Check sheet for the modelled part. Datum: model origin and axes. Units: mm. Face numbers are marked on the shaded views. Give positions to 0.01 mm unless a question says otherwise; leave off trailing zeros. Loops run counter-clockwise (first coordinate to the right, second up) from the corner with the lowest first, then second, coordinate; pieces in that order, holes last.
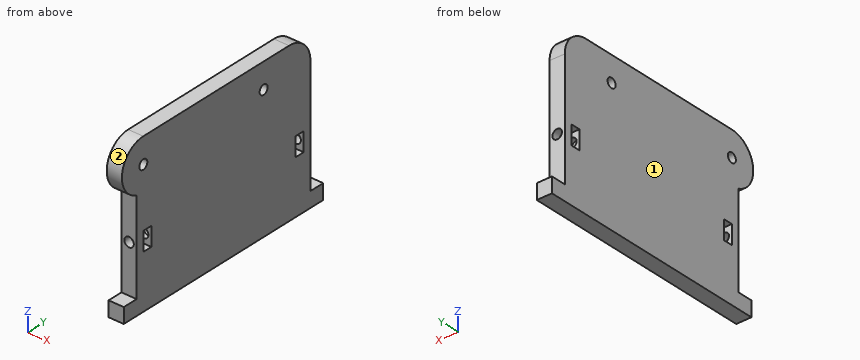
Autodesk Fusion 360 part; units mm, degrees
sketch "Sketch1" plane through (0, 0, 0) normal (1, 0, 0) x (0, 1, 0)
  line L0 (-32.5, 4.8) -> (-37.3, 4.8)
  line L1 (-37.3, 4.8) -> (-37.3, 0)
  line L2 (-37.3, 0) -> (37.3, 0)
  line L3 (37.3, 0) -> (37.3, 4.8)
  line L4 (37.3, 4.8) -> (32.5, 4.8)
  line L5 (-32.5, 4.8) -> (-32.5, 34.2007)
  line L6 (-30, 49.8) -> (24.5, 49.8)
  line L7 (32.5, 41.8) -> (32.5, 4.8)
  line L8 (-30, 41.8) -> (15, 41.8) construction
  circle A0 centre (-30, 41.8) radius 1.5
  line L9 (15, 41.8) -> (24.5, 41.8) construction
  arc A1 (24.5, 49.8) -> (32.5, 41.8) centre (24.5, 41.8) ccw construction
  arc A2 (32.5, 41.8) -> (24.5, 49.8) centre (24.5, 41.8) ccw
  line L10 (24.5, 49.8) -> (32.5, 49.8) construction
  line L11 (32.5, 49.8) -> (32.5, 41.8) construction
  circle A3 centre (15, 41.8) radius 1.5
  circle A4 centre (-25, 41.8) radius 5 construction
  circle A5 centre (25, 41.8) radius 5 construction
  line L12 (-25, 41.8) -> (25, 41.8) construction
  line L13 (0, 41.8) -> (0, 0) construction
  arc A6 (-32.5, 34.2007) -> (-30, 49.8) centre (-30, 41.8) ccw construction
  arc A7 (-30, 49.8) -> (-32.5, 34.2007) centre (-30, 41.8) ccw
  point P0 (0, 41.8)
  dimension "d1" = 4.8
  dimension "d2" = 4.8
  dimension "d3" = 74.6
  dimension "d4" = 4.8
  dimension "d5" = 4.8
  dimension "d6" = 45
  dimension "d8" = 45
  dimension "d9" = 8
  dimension "d11" = 3
  dimension "d12" = 16
  dimension "d13" = 3
  dimension "d14" = 10
  dimension "d15" = 10
  dimension "d16" = 50
  dimension "d17" = 10
extrude "Extrude1" add sketch "Sketch1" along normal blind 4.8
sketch "Sketch2" plane through (0, -32.5, 0) normal (0, -1, 0) x (1, 0, 0)
  line L0 (0, 34.2007) -> (0, 4.8)
  line L1 (0, 4.8) -> (4.8, 4.8)
  line L2 (4.8, 4.8) -> (4.8, 34.2007)
  line L3 (4.8, 34.2007) -> (0, 34.2007)
  line L4 (0, 4.8) -> (0, 0)
  line L5 (0, 0) -> (4.8, 0)
  line L6 (4.8, 0) -> (4.8, 4.8)
  line L7 (4.8, 4.8) -> (0, 4.8)
  circle A0 centre (2.4, 20) radius 1.5
  dimension "d20" = 3
  dimension "d21" = 20
  dimension "d22" = 2.4
hole "Hole1" at (2.4, -32.5, 20) direction (0, 1, 0) diameter 3 depth 7.2 tip angle 118
sketch "Sketch3" plane through (0, 32.5, 0) normal (0, 1, 0) x (-1, 0, 0)
  line L0 (0, 4.8) -> (0, 41.8)
  line L1 (0, 41.8) -> (-4.8, 41.8)
  line L2 (-4.8, 41.8) -> (-4.8, 4.8)
  line L3 (-4.8, 4.8) -> (0, 4.8)
  line L4 (0, 0) -> (0, 4.8)
  line L5 (0, 4.8) -> (-4.8, 4.8)
  line L6 (-4.8, 4.8) -> (-4.8, 0)
  line L7 (-4.8, 0) -> (0, 0)
  circle A0 centre (-2.4, 20) radius 1.5
  dimension "d26" = 3
  dimension "d27" = 20
  dimension "d28" = 2.4
hole "Hole2" at (2.4, 32.5, 20) direction (0, -1, 0) diameter 3 depth 7.2 tip angle 118
sketch "Sketch4" plane through (4.8, 0, 0) normal (1, 0, 0) x (0, 1, 0)
  circle A0 centre (15, 41.8) radius 1.5
  circle A1 centre (-30, 41.8) radius 1.5
  arc A2 (32.5, 41.8) -> (24.5, 49.8) centre (24.5, 41.8) ccw
  line L0 (24.5, 49.8) -> (-30, 49.8)
  arc A3 (-30, 49.8) -> (-32.5, 34.2007) centre (-30, 41.8) ccw
  line L1 (-32.5, 34.2007) -> (-32.5, 4.8)
  line L2 (-32.5, 4.8) -> (-37.3, 4.8)
  line L3 (-37.3, 4.8) -> (-37.3, 0)
  line L4 (-37.3, 0) -> (37.3, 0)
  line L5 (37.3, 0) -> (37.3, 4.8)
  line L6 (37.3, 4.8) -> (32.5, 4.8)
  line L7 (32.5, 4.8) -> (32.5, 41.8)
  line L8 (-32.5, 18.5) -> (-25.3, 18.5) construction
  line L9 (-25.3, 18.5) -> (-25.3, 21.5) construction
  line L10 (-25.3, 21.5) -> (-32.5, 21.5) construction
  line L11 (32.5, 21.5) -> (25.3, 21.5) construction
  line L12 (25.3, 21.5) -> (25.3, 18.5) construction
  line L13 (25.3, 18.5) -> (32.5, 18.5) construction
  line L14 (-25.3, 20) -> (25.3, 20) construction
  line L15 (-30, 17) -> (-27, 17)
  line L16 (-27, 17) -> (-27, 23)
  line L17 (-27, 23) -> (-30, 23)
  line L18 (-30, 23) -> (-30, 17)
  line L19 (-25.3, 20) -> (-27, 20) construction
  line L20 (27, 23) -> (30, 23)
  line L21 (30, 23) -> (30, 17)
  line L22 (30, 17) -> (27, 17)
  line L23 (27, 17) -> (27, 23)
  line L24 (27, 20) -> (25.3, 20) construction
  point P0 (-25.3, 20)
  point P1 (25.3, 20)
  point P2 (-27, 20)
  point P3 (27, 20)
  dimension "d32" = 7.2
  dimension "d33" = 3
  dimension "d34" = 7.2
  dimension "d35" = 3
  dimension "d36" = 20
  dimension "d37" = 3
  dimension "d38" = 6
  dimension "d39" = 2.5
  dimension "d40" = 3
  dimension "d41" = 6
  dimension "d42" = 2.5
extrude "Extrude2" cut sketch "Sketch4" against normal through all contours L15 L16 L17 L18 | L20 L21 L22 L23
(1) Material ranges on line 1 (Y direction, x = 1.7, z = 22); line 2 (Y direction, x = 3.95, z = 41); line 3 (Z direction, x = 3.35, y = 15), recorded low to high.
(2) Release check for a two-part mould opening along Z. For the marked faces 1 and 2 record: pulls with the +Z half, pulls with the -Z half, needs draft (parallel to the pull), parting line crosses it, or undercut.
(3) Section check D-D on z = 31.5. Record the boundary of the cut face in (x, y).
(4) Section check C-C on x = 3.15. Give the number of separate pieces and of enclosed holes in the cut face, plus the area to 3 significant figures.
(5) Gauge pin test, flat ends, axial feed: pin 1 Ø1.5 at (y, z) = (-21.5, 33) entering from -X; pin 2 Ø2.5 at (x, z) = (2.4, 20) entering from +Y; pin 3 Ø2 at (x, z) = (1, 8.5) entering from -Y; pin 4 Ø1.4 at (x, z) = (1.5, 2.5) entering from -Y. Record the tip position at first contact, or that the pin passes through.
(6) Section check A-A on y = 15. Record the boundary of the cut face in (x, z), plus the area to 3 significant figures.
(7) Section check B-B on y = 33.5. Record the boundary of the cut face in (x, z).
Computed values:
1. line 1: y = -32.5 to -30, -27 to 27, 30 to 32.5
1. line 2: y = -37.96 to -31.27, -28.73 to 13.73, 16.27 to 32.5
1. line 3: z = 0 to 40.3, 43.3 to 49.8
2. face 1: needs draft
2. face 2: undercut
3. outline: (0, -32.5) - (4.8, -32.5) - (4.8, 32.5) - (0, 32.5) - close
4. separate pieces: 1
4. enclosed holes: 2
4. area: 3,260 mm2
5. pin 1: stops at x = 0
5. pin 2: stops at y = 25.15
5. pin 3: stops at y = -32.5
5. pin 4: stops at y = -37.3
6. outline: (0, 0) - (4.8, 0) - (4.8, 40.3) - (0, 40.3) - close; (0, 43.3) - (4.8, 43.3) - (4.8, 49.8) - (0, 49.8) - close
6. area: 225 mm2
7. outline: (0, 0) - (4.8, 0) - (4.8, 4.8) - (0, 4.8) - close
